Build history of the part. All positions in model axes, mm. A direction names the side the tool comes from. Give positions to 0.01 mm unless a question says otherwise; leave off trailing zeros. Order: outer loops, then holes, each group sorted by start corner. A loop starts at its lowest first (then second) coordinate and runs counter-clockwise, first axis right, second up. Notation, with made-up numbers: (9.25, 33.25) -> (35.25, 33.25) arc R5 ccw to (35.25, 41.25) -> close; hole circle Ø11 at (10.25, 21). An arc over 180 degrees is marked (long way). One line per item, written item: value. Start each with the question number.
(1) Two-plate mould, pull along X, no slides. Class faces 1 (the flat face through (-1, -63.5, 0)), 2 (the flat face through (41.275, -1, 4)), 3 (the cylindrical face through (45.8, -0.4, 38.1)): +X half, -X half, draft (parallel to the pull), parting line (faces both ways), or undercut.
(2) Probe line 1 (Z direction, x = 81.5, y = 22.5) (3 decimals); line 2 (Y direction, x = 41, z = 33.5); line 3 (X direction, y = -20, z = 2.5) (3 decimals). List the from-to ranges inside material, lowest first.
(3) Saw through at B-B on x = 88. Give the cut face in (y, z) (3 decimals).
(4) Which spindle directions (+Z, -Z, +X, -X, +Y, -Y) get a long thin tool onto all of the face, cutting with end or side? Do faces 4 (the flat face through (60, -2, 61.925)), 5 (the flat face through (-5, 7.938, 30)), 6 (the flat face through (46, -25.4, 42)), 7 (the flat face through (22.225, -17, 18)). Say none if no direction does.
(5) Pin check, flat tips, straight feed: pin 1 (4 mm diameter, centred on x = 28, y = 44.5, fed in from +Z) (3 decimals); pin 2 (2 mm diameter, centred on x = 64, y = 11.5, fed in from -Z); pin 3 (2 mm diameter, centred on x = 16, z = 24.5, fed in from +Y). Stop position of each tip, or through.
(6) Saw through at A-A on y = -48. Give the cut face in (x, z) (3 decimals), plus the area to 3 significant figures.
```python
from build123d import *

# Parameters (mm, degrees)
F1_DEPTH = 63.5
F0_W     = 25.4
F0_H     = 19.05
F2_DEPTH = 25.4
F3_DEPTH = 7.9375


with BuildPart() as f1:
    # F0 (on Front) → F1 (new body, symmetric)
    with BuildSketch(Plane.XZ):
        Polygon((41.275, -9.525), (41.275, 9.525), (22.225, 9.525), (-41.275, 9.525), (-41.275, -9.525), align=None)
    extrude(amount=F1_DEPTH, both=True)

    # F0 (on Front) → F2 (join, symmetric)
    with BuildSketch(Plane.XZ):
        with Locations((73.025, 52.4002)):
            Rectangle(F0_W, F0_H)
        with BuildLine():
            Line((22.225, 9.525), (41.275, 9.525))
            Line((41.275, 9.525), (41.275, 27.0002))
            ThreePointArc((41.275, 27.0002), (45.9246798487, 38.2255201513), (57.15, 42.8752))
            Line((57.15, 42.8752), (60.325, 42.8752))
            Line((60.325, 42.8752), (60.325, 61.9252))
            Line((60.325, 61.9252), (57.15, 61.9252))
            add(Edge.make_bspline(
                [(54.7396282089, 61.841924022), (55.5498180251, 61.8762426879), (56.3534740618, 61.9040043012), (57.15, 61.9252)],
                knots=[109.298641458, 109.298641458, 109.298641458, 109.298641458, 111.5045361635, 111.5045361635, 111.5045361635, 111.5045361635], degree=3))
            ThreePointArc((54.7396282089, 61.841924022), (31.6163177371, 50.828475118), (22.225, 27.0002))
            Line((22.225, 27.0002), (22.225, 9.525))
        make_face()
    extrude(amount=F2_DEPTH, both=True)

    # F0 (on Front) → F3 (join, symmetric)
    with BuildSketch(Plane.XZ):
        with BuildLine():
            Line((-41.275, 9.525), (22.225, 9.525))
            Line((22.225, 9.525), (22.225, 27.0002))
            ThreePointArc((22.225, 27.0002), (31.6163177371, 50.828475118), (54.7396282089, 61.841924022))
            add(Edge.make_bspline(
                [(-41.275, 9.525), (-41.5883963276, 42.3431733754), (14.595986714, 60.1414876679), (54.7396282089, 61.841924022)],
                knots=[0, 0, 0, 0, 109.298641458, 109.298641458, 109.298641458, 109.298641458], degree=3))
        make_face()
    extrude(amount=F3_DEPTH, both=True)

    # F0 (on Front) → F4 (revolve)
    with BuildSketch(Plane.XZ):
        Polygon((85.725, 61.9252), (85.725, 42.8752), (85.725, 38.1), (111.125, 38.1), (111.125, 66.675), (85.725, 66.675), align=None)
    revolve(axis=Axis((85.725, 0, 52.3875), (0, 0, 1)))


solid = f1.part
```
Results below:
1. face 1: draft
1. face 2: +X half
1. face 3: undercut
2. line 1: z = 38.1 to 66.675
2. line 2: y = -25.4 to 25.4
2. line 3: x = -41.275 to 41.275
3. outline: (-25.298, 38.1) -> (25.298, 38.1) -> (25.298, 66.675) -> (-25.298, 66.675) -> close
4. face 4: +Z, -X
4. face 5: +Z, -X, +Y
4. face 6: +Z, +X, -X, -Y
4. face 7: +Z, -X, -Y
5. pin 1: stops at z = 9.525
5. pin 2: stops at z = 38.1
5. pin 3: stops at y = 7.94
6. outline: (-41.275, -9.525) -> (41.275, -9.525) -> (41.275, 9.525) -> (-41.275, 9.525) -> close
6. area: 1,570 mm²
